Input: dimensioned drawing with shaded views. Units: mm. Origin: part minimum x, y, z. Give positions to 0.01 mm unless a question says otherwise; leave off trailing zeros. Loops run counter-clockwise (first coordinate to the right, second up) from the corner with the lowest first, then second, coordinate; pieces in that order, holes last. Notation, with made-up numbers: (16.25, 45.5) -> (32.25, 45.5) arc R27 cw to (32.25, 78.5) -> close; hole circle Ø11 at (14, 13). An arc over 180 degrees is marked (long way). Answer in a Markdown table with one row per item. Add a question column.
1) First-contact query: P1, Ø4, axis at x = 1.5, z = 38, coming from the +Y side; P2, Ø1, axis at x = 5, z = 150.5, coming from the -Y side. Flat tips, straight axial feed; report the tip coordinate or a pass-through.
2) Section query B-B (y = 6.25). Return the cut outline in (x, z), plus the area to 3 significant figures.
3) Line query: line 1 (X direction, y = 3.5, z = 182); line 2 (Y direction, x = 3, z = 53). Output: solid intervals per line, ascending. Write a range as from..to.
4) Section query A-A (z = 27.5). Return the cut outline in (x, y).
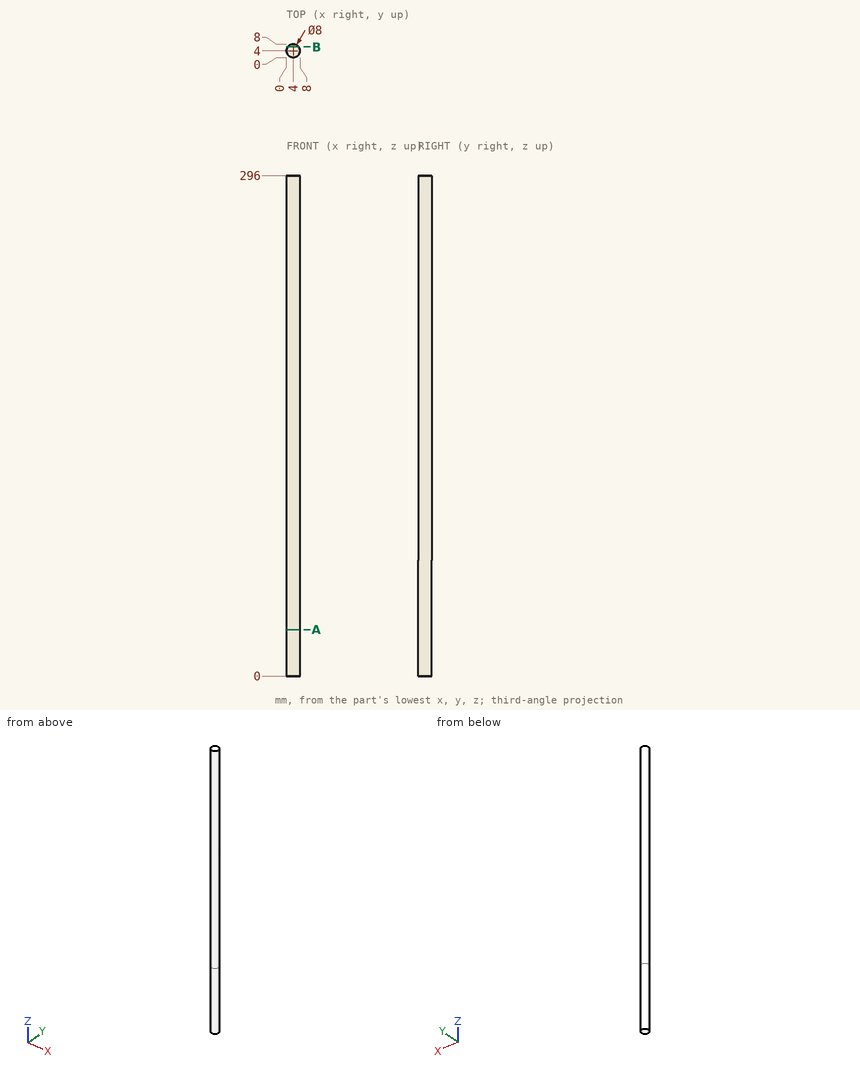
Evaluation:
| question | item | result |
|---|---|---|
| 1 | P1 | y = 7.97 |
| 1 | P2 | y = 0.03 |
| 2 | outline | (0.69, 0) -> (7.31, 0) -> (7.31, 296) -> (0.69, 296) -> close |
| 2 | area | 1,960 mm² |
| 3 | line 1 | 0.03..7.97 |
| 3 | line 2 | 0.13..7.87 |
| 4 | outline | circle Ø8 at (4, 4) |
